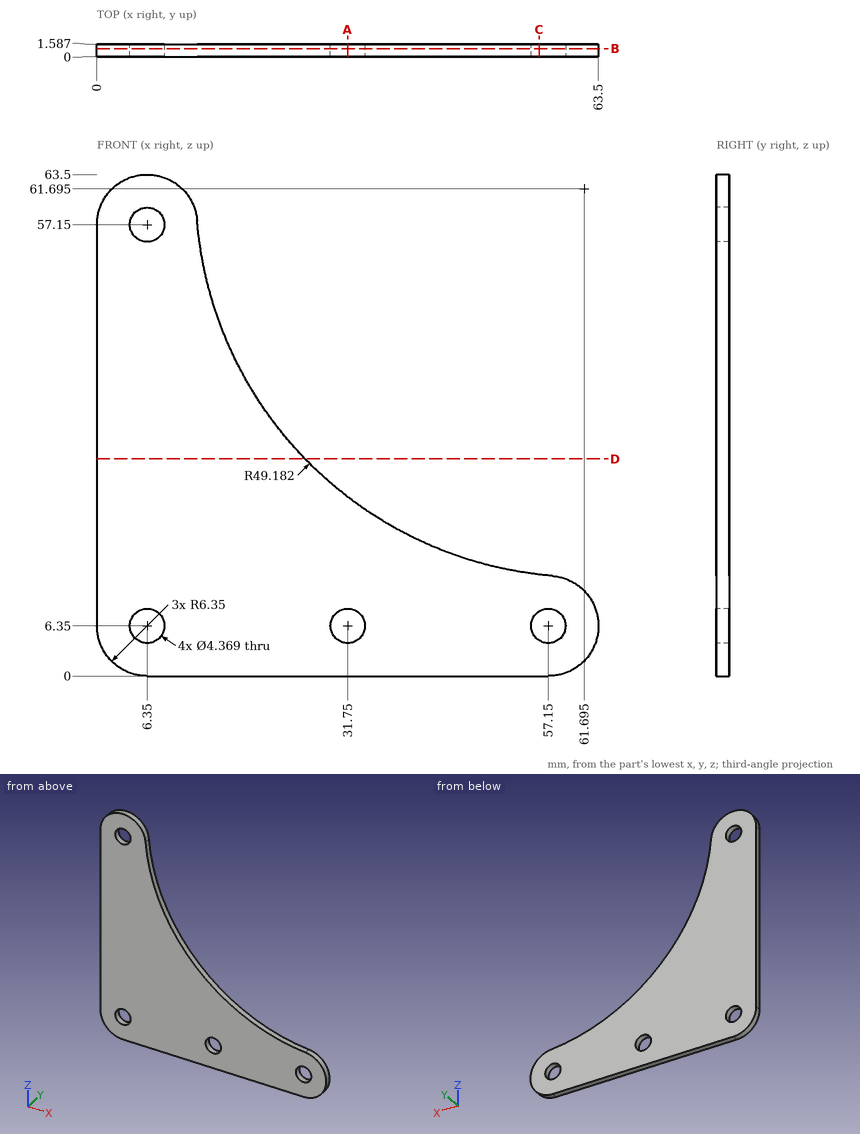
For this review, use the dimensioned drawing (mm, ordinates from the lowest corner) and the shaded views. Give positions to 0.01 mm unless a question says otherwise; leave off trailing zeros. Order: outer loops, then holes, each group sorted by start corner. A loop starts at its lowest first (then second) coordinate and runs counter-clockwise, first axis right, second up. Notation, with made-up numbers: (25.25, 78.5) - (66.25, 78.5) arc R37 cw to (66.25, 115.5) - close; hole circle Ø6 at (5.5, 51). An arc over 180 degrees is marked (long way). Write item = value, one per line. Start each with the question number.
Q1. We need section D-D on z = 27.5. State the section outline as (x, y) points.
Q2. We need section A-A on x = 31.75. State the section outline as (y, z) points (1 decimal).
Q3. We need section B-B on y = 1. State how many separate pieces and enclosed holes the cut face has, plus the area to 3 significant figures.
Q4. To check wall thickness, follow L1, parallel to Z at x = 6.35, y = 0.9 (1 decimal); L2, parallel to X at y = 1, z = 8 (1 decimal); L3, parallel to Z at x = 33.5, y = 0.45 (1 decimal). State the ranges of each line that lie inside material, in increasing order. Write a range as from..to.
Q5. We need section C-C on x = 56. State the section outline as (y, z) points (1 decimal), plus the area to 3 significant figures.
Working result:
q1.outline = (0, 0) - (26.35, 0) - (26.35, 1.59) - (0, 1.59) - close
q2.outline = (0, 0) - (1.6, 0) - (1.6, 4.2) - (0, 4.2) - close; (0, 8.5) - (1.6, 8.5) - (1.6, 22.7) - (0, 22.7) - close
q3.separate_pieces = 1
q3.enclosed_holes = 4
q3.area = 1,850 mm²
q4.L1 = 0..4.2, 8.5..55, 59.3..63.5
q4.L2 = 0..4.9, 7.8..30.3, 33.2..55.7, 58.6..63.3
q4.L3 = 0..5, 7.7..21.4
q5.outline = (0, 0) - (1.6, 0) - (1.6, 4.5) - (0, 4.5) - close; (0, 8.2) - (1.6, 8.2) - (1.6, 12.8) - (0, 12.8) - close
q5.area = 14.5 mm²
